Input: part model. Units: mm. Frame: model coordinates. Give positions to 0.01 mm unless a question says otherwise; leave off trailing zeros. Loops run counter-clockwise (first coordinate to the right, second up) from the corner with the lowest first, then second, coordinate; pieces in that order, holes last. Notation, with made-up numbers: M -17,46 L 3,46 A23 cw 3,68 Z; hole C 35,0.25 d3. An arc over 180 degrees is marked long. One line per item, written item: value. Start each with the question number.
(1) Section A-A on z = -36.5. Output: boundary loops of the cut face in (x, y) (3 decimals), plus the area to 3 significant figures.
(2) Section B-B on y = 13. Output: boundary loops of the cut face in (x, z) (3 decimals), plus the area to 3 significant figures.
(3) Ray query, line 1 along Z through (x, y) = (1.65, 8.5); line 2 along Y through (x, z) = (3.05, -38); line 3 along Y through (x, z) = (2.8, 8.5). Return the intervals inside material, ascending. Write a range as from..to.
(4) Section C-C on z = -5. Output: boundary loops of the cut face in (x, y) (3 decimals), plus the area to 3 significant figures.
(5) Pin query (flat end, axial travel): P1, Ø1, axis at y = 21.5, z = -42, coming from the -X side; P2, Ø1, axis at x = 1.5, z = -1, coming from the -Y side; P3, Ø1.5, axis at x = 1, y = -10, coming from the -Z side; P4, Ø1, axis at x = 2, y = -29, coming from the +Z side. Return the tip coordinate at first contact, or that it passes through.
(6) Section D-D on x = 0.75. State how many separate pieces and enclosed holes the cut face has, plus the area to 3 significant figures.
Autodesk Inventor part; units mm, degrees
ref_plane "YZ Plane" through (0, 0, 0) normal (1, 0, 0) x (0, 1, 0)
ref_plane "XZ Plane" through (0, 0, 0) normal (0, 1, 0) x (-1, 0, 0)
ref_plane "XY Plane" through (0, 0, 0) normal (0, 0, 1) x (1, 0, 0)
sketch "Sketch1" plane through (0, 0, 0) normal (1, 0, 0) x (0, 1, 0)
  line L0 (33.2271, 21.6336) -> (-27.7329, 21.6336)
  line L1 (-27.7329, 21.6336) -> (-27.7329, -50.7564)
  line L2 (-27.7329, -50.7564) -> (33.2271, -50.7564)
  line L3 (33.2271, -50.7564) -> (33.2271, 21.6336)
  line L4 (33.2271, -38.0564) -> (36.4021, -38.0564)
  line L5 (36.4021, -38.0564) -> (36.4021, -29.1664)
  line L6 (36.4021, -29.1664) -> (33.2271, -29.1664)
  line L7 (33.2271, -29.1664) -> (33.2271, -38.0564)
  line L8 (33.2271, 8.9336) -> (36.4021, 8.9336)
  line L9 (36.4021, 8.9336) -> (36.4021, 0.0436)
  line L10 (36.4021, 0.0436) -> (33.2271, 0.0436)
  line L11 (33.2271, 0.0436) -> (33.2271, 8.9336)
  line L12 (33.2271, -16.4664) -> (36.4021, -16.4664)
  line L13 (36.4021, -16.4664) -> (36.4021, -12.6564)
  line L14 (36.4021, -12.6564) -> (33.2271, -12.6564)
  line L15 (33.2271, -12.6564) -> (33.2271, -16.4664)
  line L16 (33.2271, 21.6336) -> (20.5271, 21.6336)
  line L17 (20.5271, 21.6336) -> (20.5271, 24.8086)
  line L18 (20.5271, 24.8086) -> (33.2271, 24.8086)
  line L19 (33.2271, 24.8086) -> (33.2271, 21.6336)
  line L20 (-27.7329, 21.6336) -> (-15.0329, 21.6336)
  line L21 (-15.0329, 21.6336) -> (-15.0329, 24.8086)
  line L22 (-15.0329, 24.8086) -> (-27.7329, 24.8086)
  line L23 (-27.7329, 24.8086) -> (-27.7329, 21.6336)
  line L24 (-4.8729, 21.6336) -> (10.3671, 21.6336)
  line L25 (10.3671, 21.6336) -> (10.3671, 24.8086)
  line L26 (10.3671, 24.8086) -> (-4.8729, 24.8086)
  line L27 (-4.8729, 24.8086) -> (-4.8729, 21.6336)
  point P0 (0, 0)
  dimension "d0" = 60.96
  dimension "d1" = 72.39
  dimension "d2" = 12.7
  dimension "d3" = 8.89
  dimension "d4" = 3.175
  dimension "d5" = 8.89
  dimension "d6" = 12.7
  dimension "d7" = 12.7
  dimension "d8" = 12.7
  dimension "d11" = 3.175
  dimension "d12" = 12.7
  dimension "d13" = 12.7
  dimension "d14" = 10.16
  dimension "d15" = 10.16
ref_plane "Work Plane1" through (0, 2.7471, 0.0436) normal (0, 1, 0) x (1, 0, 0)
extrude "Extrusion3" add sketch "Sketch1" along normal blind 3.175
ref_plane "Work Plane2" through (0, -15.0329, -14.5614) normal (0, 0, 1) x (1, 0, 0)
mirror "Mirror2" about plane through (0, -15.0329, -14.5614) normal (0, 0, 1) of "Extrusion3"
mirror "Mirror3" about plane through (0, 2.7471, 0.0436) normal (0, 1, 0) of "Extrusion3"
sketch "Sketch2" plane through (0, 0, 0) normal (-1, 0, 0) x (0, 0, 1)
  line L0 (-40.3424, -22.1449) -> (-31.1984, -22.1449)
  line L1 (-31.1984, -22.1449) -> (-31.1984, -10.7149)
  line L2 (-31.1984, -10.7149) -> (-40.3424, -10.7149)
  line L3 (-40.3424, -10.7149) -> (-40.3424, -22.1449)
  line L4 (-38.0564, -30.9079) -> (-29.1664, -30.9079)
  line L5 (-50.7564, -15.0329) -> (-50.7564, -4.8729)
  point P0 (0, 0)
  dimension "d20" = 20.193
  dimension "d21" = 11.43
  dimension "d22" = 9.144
  dimension "d23" = 10.414
extrude "Extrusion4" cut sketch "Sketch2" against normal blind 3.175
sketch "Sketch3" plane through (0, 0, 0) normal (-1, 0, 0) x (0, 0, 1)
  line L0 (-38.0564, 8.0811) -> (8.9336, 8.0811)
  line L1 (8.9336, 8.0811) -> (8.9336, 15.7011)
  line L2 (8.9336, 15.7011) -> (-38.0564, 15.7011)
  line L3 (-38.0564, 15.7011) -> (-38.0564, 8.0811)
  line L4 (-16.4664, -27.7329) -> (-29.1664, -27.7329)
  line L5 (-50.7564, 10.3671) -> (-50.7564, 20.5271)
  line L6 (21.6336, 20.5271) -> (21.6336, 10.3671)
  line L7 (-20.9114, 8.0811) -> (-8.2114, 8.0811)
  line L8 (-8.2114, 8.0811) -> (-8.2114, 15.7011)
  line L9 (-8.2114, 15.7011) -> (-20.9114, 15.7011)
  line L10 (-20.9114, 15.7011) -> (-20.9114, 8.0811)
  point P0 (0, 0)
  dimension "d26" = 43.434
  dimension "d27" = 7.62
  dimension "d28" = 12.7
  dimension "d29" = 12.7
  dimension "d30" = 12.7
  dimension "d31" = 46.99
  dimension "d32" = 17.145
  dimension "d33" = 17.145
extrude "Extrusion5" cut sketch "Sketch3" against normal blind 3.175 contours L3 L2 L10 L0 | L8 L2 L1 L0
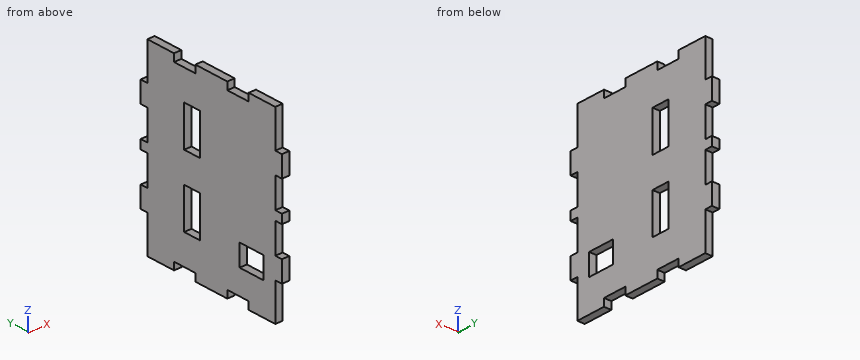
Output values:
1. outline: M 0,-30.908 L 3.175,-30.908 L 3.175,-22.145 L 0,-22.145 Z; M 0,-10.715 L 3.175,-10.715 L 3.175,8.081 L 0,8.081 Z; M 0,15.701 L 3.175,15.701 L 3.175,36.402 L 0,36.402 Z
1. area: 153 mm²
2. outline: M 0,-50.756 L 3.175,-50.756 L 3.175,-38.056 L 0,-38.056 Z; M 0,-20.911 L 3.175,-20.911 L 3.175,-8.211 L 0,-8.211 Z; M 0,8.934 L 3.175,8.934 L 3.175,21.634 L 0,21.634 Z
2. area: 121 mm²
3. line 1: z = -53.93..-38.06, -20.91..-8.21, 8.93..24.81
3. line 2: y = -30.91..-22.14, -10.71..8.08, 15.7..36.4
3. line 3: y = -30.91..8.08, 15.7..36.4
4. outline: M 0,-27.733 L 3.175,-27.733 L 3.175,8.081 L 0,8.081 Z; M 0,15.701 L 3.175,15.701 L 3.175,33.227 L 0,33.227 Z
4. area: 169 mm²
5. P1: stops at x = 0
5. P2: stops at y = -27.73
5. P3: stops at z = -50.76
5. P4: stops at z = 8.93
6. separate pieces: 1
6. enclosed holes: 3
6. area: 4,440 mm²
